Model file for the job. Use its own axes, mm. Round coordinates to 2 decimals unless told otherwise and drop trailing zeros.
from build123d import *

# Parameters (mm, degrees)
F0_W     = 300
F0_H     = 24.5
F0_R     = 2.65
F1_DEPTH = 2
F2_DEPTH = 10
F3_DEPTH = 30
F4_R     = 1.7
F5_DEPTH = 2
F6_R     = 1.25
F7_DEPTH = 2


with BuildPart() as f1:
    # F0 (on Top) → F1 (new body)
    with BuildSketch(Plane.XY):
        Rectangle(F0_W, F0_H)
        with Locations((-45, 0)):
            Circle(F0_R, mode=Mode.SUBTRACT)
        with Locations((-30, 0)):
            Circle(F0_R, mode=Mode.SUBTRACT)
        with Locations((-15, 0)):
            Circle(F0_R, mode=Mode.SUBTRACT)
        Circle(F0_R, mode=Mode.SUBTRACT)
        with Locations((15, 0)):
            Circle(F0_R, mode=Mode.SUBTRACT)
        with Locations((30, 0)):
            Circle(F0_R, mode=Mode.SUBTRACT)
        with Locations((45, 0)):
            Circle(F0_R, mode=Mode.SUBTRACT)
    extrude(amount=F1_DEPTH)

    # F2 (add): a face of the model
    f2_faces = [f1.faces().sort_by_distance(p)[0] for p in [
        (-150, 0, 1),
    ]]
    extrude(f2_faces, amount=F2_DEPTH)

    # F3 (add): a face of the model
    f3_faces = [f1.faces().sort_by_distance(p)[0] for p in [
        (150, 0, 1),
    ]]
    extrude(f3_faces, amount=F3_DEPTH)

    # F4 (on face) → F5 (cut, through all)
    with BuildSketch(Plane.XY.offset(2)):
        with Locations((-153.6, 0)):
            Circle(F4_R)
    extrude(amount=-F5_DEPTH, mode=Mode.SUBTRACT)

    # F6 (on face) → F7 (cut, through all)
    with BuildSketch(Plane.XY.offset(2)):
        with Locations((158.75, -7.25)):
            Circle(F6_R)
    extrude(amount=-F7_DEPTH, mode=Mode.SUBTRACT)


solid = f1.part
Q1. Slice it at A-A on z = 1.55. State how many separate pieces and enclosed holes the cut face has, plus the area to 3 significant figures.
Q2. Probe line 1 (Y direction, x = -15, z = 0.8); line 2 (Y direction, x = 158.75, z = 0.7); line 3 (X direction, y = -6.25, z = 1.45). List the from-to ranges inside material, lowest first.
Q3. Pull direction X, two halves, no side cores. Call faces 1 (the face through (-47.647, 0.117, 0.986)), 2 (the face through (8, 0, 0)): pulls with the +X half, pulls with the -X half, needs draft (parallel to the pull), parting line crosses it, or undercut.
Reply:
1. separate pieces: 1
1. enclosed holes: 9
1. area: 8,160 mm2
2. line 1: y = -12.25 to -2.65, 2.65 to 12.25
2. line 2: y = -12.25 to -8.5, -6 to 12.25
2. line 3: x = -160 to 158, 159.5 to 180
3. face 1: undercut
3. face 2: needs draft
